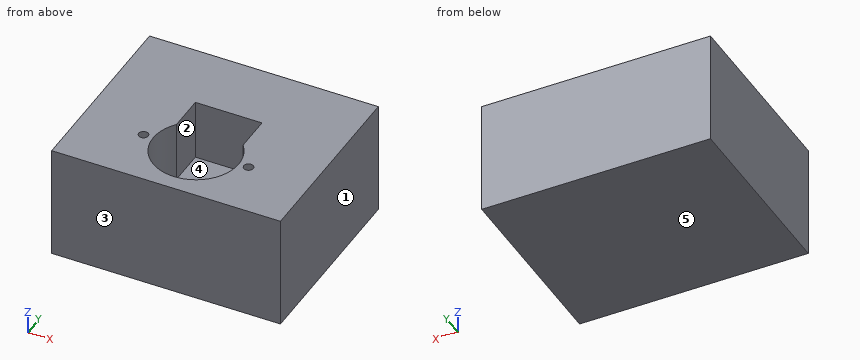
from build123d import *

# Parameters (mm, degrees)
SKETCH1_W           = 76.2
SKETCH1_H           = 63.5
BOSS_EXTRUDE1_DEPTH = 38.1
CUT_EXTRUDE2_DEPTH  = 20.32
SKETCH6_R           = 1.58
CUT_EXTRUDE3_DEPTH  = 20.32


with BuildPart() as part:
    # Sketch1 → Boss-Extrude1 (new body)
    with BuildSketch(Plane.XY):
        Rectangle(SKETCH1_W, SKETCH1_H)
    extrude(amount=BOSS_EXTRUDE1_DEPTH)

    # Sketch5 → Cut-Extrude2 (cut)
    with BuildSketch(Plane.XY.offset(38.1)):
        with BuildLine():
            Line((-11.095417071, -3.367534501), (-11.095417071, 8.870920326))
            Line((-11.095417071, 8.870920326), (11.095417071, 8.870920326))
            Line((11.095417071, 8.870920326), (11.095417071, -3.367534501))
            ThreePointArc((11.095417071, -3.367534501), (0, -26.569619951), (-11.095417071, -3.367534501))
        make_face()
    extrude(amount=-CUT_EXTRUDE2_DEPTH, mode=Mode.SUBTRACT)

    # Sketch6 → Cut-Extrude3 (cut)
    with BuildSketch(Plane.XY.offset(38.1)):
        with Locations((17.5, -12.315620011)):
            Circle(SKETCH6_R)
        with Locations((-17.5, -12.315620011)):
            Circle(SKETCH6_R)
    extrude(amount=-CUT_EXTRUDE3_DEPTH, mode=Mode.SUBTRACT)


solid = part.part
Could you check a few things on this model? Use its own coordinates, in mm. Face numbers are marked on the shaded views. A direction names the side the tool comes from. Give positions to 0.01 mm unless a question says otherwise; leave off trailing zeros. Order: outer loops, then holes, each group sorted by start corner. A loop starts at its lowest first (then second) coordinate and runs counter-clockwise, first axis right, second up. Notation, with made-up numbers: (-21, -13) - (13, -13) arc R8 ccw to (13, -5) - close; hole circle Ø3 at (60, -20.75). An arc over 180 degrees is marked (long way). One line per question, with ' | ' between items. Start each with the question number.
Item 1: I want a section at B-B on z = 31. Write out the boundary of the cut face in (x, y).
Item 2: Thinking about a two-plate mould opening in X: for the marked faces 1, 2 and 3, which applies, pulls with the +X half, pulls with the -X half, needs draft (parallel to the pull), parting line crosses it, or undercut?
Item 3: I want a section at A-A on y = 5. Write out the boundary of the cut face in (x, z), then the cut area to 3 significant figures.
Item 4: I'm going to push a flat-ended pin straight in: pin 1 Ø14.5 at (x, y) = (3.5, -1.5) entering from +Z. Where does the tip first touch, or does it pass through?
Item 5: For the marked faces 4 and 5, which set-ups out of +Z, -Z, +X, -X, +Y, -Y let a thin tool reach every point of the face, with its end or its side?
Item 6: I want a section at C-C on x = 0. Write out the boundary of the cut face in (y, z).
Item 7: I need wall thicknesses on probe 1 along X at (y, z) = (-13, 18.5); probe 2 along X at (y, z) = (-2, 19.5); probe 3 along Y at (x, z) = (17.5, 33.75). Which ranges of each line are inside material? Lowest first, please. Write a range as [from, to].
Verdict:
1) outline: (-38.1, -31.75) - (38.1, -31.75) - (38.1, 31.75) - (-38.1, 31.75) - close; hole circle Ø3.16 at (-17.5, -12.32); hole (-11.1, -3.37) arc R14.25 ccw (long way) to (11.1, -3.37) - (11.1, 8.87) - (-11.1, 8.87) - close; hole circle Ø3.16 at (17.5, -12.32)
2) face 1: pulls with the +X half | face 2: undercut | face 3: needs draft
3) outline: (-38.1, 0) - (38.1, 0) - (38.1, 38.1) - (11.1, 38.1) - (11.1, 17.78) - (-11.1, 17.78) - (-11.1, 38.1) - (-38.1, 38.1) - close | area: 2,450 mm^2
4) pin 1: z = 17.78
5) face 4: +Z | face 5: -Z, +X, -X, +Y, -Y
6) outline: (-31.75, 0) - (31.75, 0) - (31.75, 38.1) - (8.87, 38.1) - (8.87, 17.78) - (-26.57, 17.78) - (-26.57, 38.1) - (-31.75, 38.1) - close
7) probe 1: [-38.1, -18.92], [-16.08, -14.24], [14.24, 16.08], [18.92, 38.1] | probe 2: [-38.1, -11.1], [11.1, 38.1] | probe 3: [-31.75, -13.9], [-10.74, 31.75]
